Source: CAD feature listing. Evaluate the final solid. Frame: model axes, mm. Give positions to 0.01 mm unless a question says otherwise; leave off trailing zeros. Order: outer loops, then holes, each group sorted by start corner. A loop starts at its lowest first (then second) coordinate and runs counter-clockwise, first axis right, second up. Notation, with made-up numbers: (8.5, -10) - (45.5, -10) arc R20 cw to (45.5, 15) - close; hole circle Ø7 at (39, 7.25). An arc over 180 degrees is marked (long way). One line per item, written item: value. Start each with the question number.
from build123d import *

# Parameters (mm, degrees)
SKETCH1_W           = 57.15
SKETCH1_H           = 25.4
BOSS_EXTRUDE1_DEPTH = 6.35
CUT_EXTRUDE1_DEPTH  = 635
SKETCH3_R           = 3.175
CUT_EXTRUDE2_DEPTH  = 6.35


with BuildPart() as part:
    # Sketch1 → Boss-Extrude1 (new body)
    with BuildSketch(Plane(origin=(0, 0, 0), x_dir=(1, 0, 0), z_dir=(0, 1, 0))):
        with Locations((28.575, 12.7)):
            Rectangle(SKETCH1_W, SKETCH1_H)
    extrude(amount=BOSS_EXTRUDE1_DEPTH)

    # Sketch2 → Cut-Extrude1 (cut)
    with BuildSketch(Plane(origin=(57.15, 0, 0), x_dir=(0, 0, -1), z_dir=(1, 0, 0))):
        with BuildLine():
            ThreePointArc((21.922541593, 0), (17.720115786, 2.9344449), (12.7, 3.96875))
            Line((12.7, 3.96875), (12.7, 0))
            Line((12.7, 0), (21.922541593, 0))
        make_face()
        with BuildLine():
            Line((12.7, 0), (12.7, 3.96875))
            ThreePointArc((12.7, 3.96875), (7.679884214, 2.9344449), (3.477458407, 0))
            Line((3.477458407, 0), (12.7, 0))
        make_face()
        with BuildLine():
            Line((21.922541593, 0), (12.7, 0))
            Line((12.7, 0), (12.7, -21.43125))
            ThreePointArc((12.7, -21.43125), (21.680256121, -17.711506121), (25.4, -8.73125))
            ThreePointArc((25.4, -8.73125), (24.498649885, -4.032115943), (21.922541593, 0))
        make_face()
        with BuildLine():
            Line((12.7, -21.43125), (12.7, 0))
            Line((12.7, 0), (3.477458407, 0))
            ThreePointArc((3.477458407, 0), (1.0343051, -13.751365786), (12.7, -21.43125))
        make_face()
    extrude(amount=-CUT_EXTRUDE1_DEPTH, mode=Mode.SUBTRACT)

    # Sketch3 → Cut-Extrude2 (cut)
    with BuildSketch(Plane(origin=(0, 6.35, 0), x_dir=(1, 0, 0), z_dir=(0, 1, 0))):
        with Locations(Location((6.35, 12.7, 0), (0, 0, 270))):
            Circle(SKETCH3_R)
        with Locations(Location((50.8, 12.7, 0), (0, 0, 270))):
            Circle(SKETCH3_R)
    extrude(amount=-CUT_EXTRUDE2_DEPTH, mode=Mode.SUBTRACT)


solid = part.part
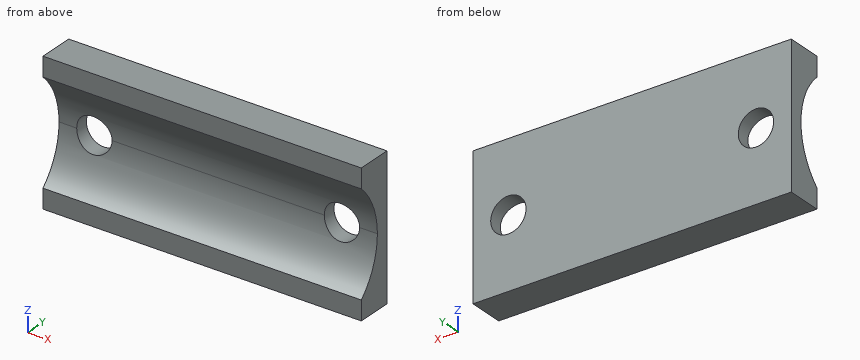
1. Section D-D on y = 5.5. Return the cut outline in (x, z) (3 decimals), then the cut area to 3 significant figures.
2. Section A-A on x = 50.8. Return the cut outline in (y, z) (3 decimals), then the cut area to 3 significant figures.
3. Ray query, L1, parallel to X at y = 5.2, z = -12.7 (3 decimals); L2, parallel to Z at x = 6.35, y = 4.5 (3 decimals); L3, parallel to X at y = 6.25, z = -11. Return the intervals inside material, ascending.
4. Section B-B on y = 2.75. Return the cut outline in (x, z), then the cut area to 3 significant figures.
5. Section C-C on z = -10.75. Return the cut outline in (x, y), then the cut area to 3 significant figures.
6. Contact query for flat-ended pins moving along their axis: pin 1 Ø2 at (x, z) = (33, -7) entering from -Y; pin 2 Ø3 at (x, z) = (43.5, -17) entering from -Y; pin 3 Ø8 at (x, z) = (26, -21) entering from -Y. Output: stop coordinate, or through.
Data:
1. outline: (0, -25.4) - (57.15, -25.4) - (57.15, 0) - (0, 0) - close; hole circle Ø6.35 at (6.35, -12.7); hole circle Ø6.35 at (50.8, -12.7)
1. area: 1,390 mm2
2. outline: (0, -25.4) - (6.35, -25.4) - (6.35, -15.875) - (3.565, -15.875) arc R12.7 cw to (0, -21.923) - close; (0, -3.477) arc R12.7 cw to (3.565, -9.525) - (6.35, -9.525) - (6.35, 0) - (0, 0) - close
2. area: 94.8 mm2
3. L1: x = 0 to 3.175, 9.525 to 47.625, 53.975 to 57.15
3. L2: z = -25.4 to -15.875, -9.525 to 0
3. L3: x = 0 to 3.67, 9.03 to 48.12, 53.48 to 57.15
4. outline: (0, -25.4) - (57.15, -25.4) - (57.15, -18.13) - (0, -18.13) - close; (0, -7.27) - (57.15, -7.27) - (57.15, 0) - (0, 0) - close
4. area: 831 mm2
5. outline: (0, 3.82) - (3.84, 3.82) - (3.84, 6.35) - (0, 6.35) - close; (8.86, 3.82) - (48.29, 3.82) - (48.29, 6.35) - (8.86, 6.35) - close; (53.31, 3.82) - (57.15, 3.82) - (57.15, 6.35) - (53.31, 6.35) - close
5. area: 119 mm2
6. pin 1: stops at y = 2.06
6. pin 2: stops at y = 2.57
6. pin 3: stops at y = 0
